Geometry check sheet. Reference: the model listing, model coordinates, mm. A direction names the side the tool comes from. Give positions to 0.01 mm unless a question says otherwise; leave off trailing zeros. Order: outer loops, then holes, each group sorted by start corner. A loop starts at its lowest first (then second) coordinate and runs counter-clockwise, first axis right, second up. Notation, with made-up numbers: M 70.5,41 L 86.5,41 A23 cw 86.5,62 Z; hole C 45,37.5 d8. An arc over 180 degrees is marked long. Put each result on its own line as item: value. Start each with the question number.
Q1. Section check C-C on y = 5. State how many separate pieces and enclosed holes the cut face has, then the cut area to 3 significant figures.
Q2. Section check A-A on z = 18. Record the cut outline in (x, y).
Q3. Go/stop test with flat-tipped pins: pin 1 (10 mm diameter, centred on x = 2.5, y = -5, fed in from -Z); pin 2 (1.5 mm diameter, centred on x = -2, y = -4.5, fed in from +Z); pin 3 (6 mm diameter, centred on x = -3.5, z = 25, fed in from -Y). Record where each tip stops, or that it passes through.
Q4. Material ranges on L1, parallel to X at y = 0, z = 38; L2, parallel to Y at x = 1.25, z = 18; L3, parallel to Y at x = 0.5, z = 28, recorded low to high.
Q5. Access from +Z, -Z, +X, -X, +Y, -Y to the whole of each face (thin tool, end or side, straight path). Record for faces 4 (the conical face through (0, 16, 1)), 5 (the cylindrical face through (-2.159, -6.856, 36.518)).
Q6. Section check B-B on z = 40. Record the cut outline in (x, y), then the cut area to 3 significant figures.
Q7. Mould release check, pull along X, two halves, no side actions. Record for faces 1 (the cylindrical face through (0.062, -7.188, 9.072)), 2 (the conical face through (0, -16, 1)), 3 (the flat face through (0, 0, 0)): +X half, -X half, draft (parallel to the pull), parting line (faces both ways), or undercut.
Autodesk Inventor part; units mm, degrees
ref_plane "YZ Plane" through (0, 0, 0) normal (1, 0, 0) x (0, 1, 0)
ref_plane "XZ Plane" through (0, 0, 0) normal (0, 1, 0) x (-1, 0, 0)
ref_plane "XY Plane" through (0, 0, 0) normal (0, 0, 1) x (1, 0, 0)
sketch "Sketch1" plane through (0, 0, 0) normal (0, 0, 1) x (1, 0, 0)
  circle A0 centre (0, 0) radius 19
  dimension "d0" = 38
extrude "Extrusion1" add sketch "Sketch1" along normal blind 48
sketch "Sketch2" plane through (0, 0, 48) normal (0, 0, 1) x (1, 0, 0)
  line L0 (12.5, 21.9531) -> (30.6636, 21.9531)
  line L1 (30.6636, 21.9531) -> (30.6636, -19.8764)
  line L2 (30.6636, -19.8764) -> (12.5, -19.8764)
  line L3 (12.5, -19.8764) -> (12.5, 21.9531)
  point P0 (0, 0)
  dimension "d3" = 12.5
extrude "Extrusion2" cut sketch "Sketch2" against normal through all
pattern_circular "Circular Pattern1" count 2 over 360 about axis through (0, 0, 0) along (0, 0, 1) of "Extrusion2"
sketch "Sketch3" plane through (12.5, -14.3091, 48) normal (1, 0, 0) x (0, 0, -1)
  circle A0 centre (30, 14.3091) radius 11
  line L0 (48, 28.6182) -> (48, 0)
  point P0 (48, 14.3091)
  point P1 (48, 14.3091)
  dimension "d9" = 22
  dimension "d10" = 18
extrude "Extrusion3" cut sketch "Sketch3" against normal through all
sketch "Sketch4" plane through (0, 0, 48) normal (0, 0, 1) x (1, 0, 0)
  arc A0 (12.5, 14.3091) -> (-12.5, 14.3091) centre (0, 0) ccw
hole "Hole1" at (0, 0, 48) direction (0, 0, -1) diameter 14.376 depth 39.3 tip angle 118
chamfer "Chamfer1" distance 4 angle 45 4 edges at (0, 19, 0) (0, -19, 0) (0, 19, 48) (0, -19, 48)
chamfer "Chamfer2" distance 1 angle 45 1 edges at (0, 7.188, 48)
chamfer "Chamfer3" distance 1 angle 45 2 edges at (12.5, 0, 29) (-12.5, 0, 29)
properties part number "IMS-01-002" material "Steel, Carbon"
Results found:
1. separate pieces: 3
1. enclosed holes: 0
1. area: 494 mm^2
2. outline: M -12.5,-14.31 A19 ccw 12.5,-14.31 L 12.5,-12 L 11.5,-11 L -11.5,-11 L -12.5,-12 Z; M -12.5,12 L -11.5,11 L 11.5,11 L 12.5,12 L 12.5,14.31 A19 ccw -12.5,14.31 Z
3. pin 1: stops at z = 0
3. pin 2: stops at z = 7.79
3. pin 3: stops at y = -18.99
4. L1: x = -12.5 to -7.19, 7.19 to 12.5
4. L2: y = -18.96 to -11, 11 to 18.96
4. L3: y = -18.99 to -7.17, 7.17 to 18.99
5. face 4: -Z, +Y
5. face 5: +Z
6. outline: M -12.5,-14.31 A19 ccw 12.5,-14.31 L 12.5,14.31 A19 ccw -12.5,14.31 Z; hole C 0,0 d14.38
6. area: 714 mm^2
7. face 1: undercut
7. face 2: parting line
7. face 3: draft
